```python
from build123d import *

# Parameters (mm, degrees)
F1_DEPTH = 70
F2_DEPTH = 2
F4_DEPTH = 25
F5_W     = 61
F5_H     = 2
F5_W_2   = 2
F6_DEPTH = 25


with BuildPart() as f1:
    # F0 (on Front) → F1 (new body)
    with BuildSketch(Plane.XZ):
        with BuildLine():
            Line((56, 11), (0, 11))
            ThreePointArc((0, 11), (-11, 0), (0, -11))
            Line((0, -11), (56, -11))
            ThreePointArc((56, -11), (67, 0), (56, 11))
        make_face()
        with BuildLine():
            ThreePointArc((0, -9.5), (-9.5, 0), (0, 9.5))
            Line((0, 9.5), (56, 9.5))
            ThreePointArc((56, 9.5), (65.5, 0), (56, -9.5))
            Line((56, -9.5), (0, -9.5))
        make_face(mode=Mode.SUBTRACT)
    extrude(amount=F1_DEPTH)

    # F0 (on Front) → F2 (join)
    with BuildSketch(Plane.XZ):
        with BuildLine():
            Line((56, 9.5), (0, 9.5))
            ThreePointArc((0, 9.5), (-9.5, 0), (0, -9.5))
            Line((0, -9.5), (56, -9.5))
            ThreePointArc((56, -9.5), (65.5, 0), (56, 9.5))
        make_face()
    extrude(amount=F2_DEPTH)

    # F3 (on face) → F4 (cut)
    with BuildSketch(Plane(origin=(0, 0, -11), x_dir=(1, 0, 0), z_dir=(0, 0, -1))):
        with BuildLine():
            Line((67, 70), (56, 70))
            Line((56, 70), (56, 68))
            ThreePointArc((56, 68), (59.221825, 60.221825), (67, 57))
            Line((67, 57), (67, 70))
        make_face()
    extrude(amount=-F4_DEPTH, mode=Mode.SUBTRACT)

    # F5 (on face) → F6 (cut)
    with BuildSketch(Plane(origin=(0, 0, -11), x_dir=(1, 0, 0), z_dir=(0, 0, -1))):
        with Locations((17.5, 36)):
            Rectangle(F5_W, F5_H)
        with Locations((67, 36)):
            Rectangle(F5_W_2, F5_H)
    extrude(amount=-F6_DEPTH, mode=Mode.SUBTRACT)


solid = f1.part
```
CAD build for the part. Positions are in the model's coordinates, mm. A direction names the side the tool comes from. Round coordinates to 2 decimals unless told otherwise and drop trailing zeros. Write each loop counter-clockwise with the first axis right and the second up, starting at its lowest first coordinate (ties: lowest second). Pieces come first, ordered by that corner, then holes. Notation, with made-up numbers: (11.25, 53) - (43.25, 53) arc R14 cw to (43.25, 78) - close; hole circle Ø8 at (76.5, 52.25). An arc over 180 degrees is marked (long way). Return JSON: item names as keys, results as strings. Group by question number.
Item 1: Probe probe 1 along Z at (x, y) = (40.5, -57); probe 2 along Y at (x, z) = (4, -9.75); probe 3 along Y at (x, z) = (36, -6.25). List the from-to ranges inside material, lowest first.
Item 2: Band-saw the part on C-C on y = -20. List the corners of the cut face in (x, z), plus the area to 3 significant figures.
Item 3: 3-axis set-ups, long thin cutter, end or side, ignore diameter. For faces 1 (the face through (66, -36, 0)), 2 (the face through (16, -35, -10)), 3 (the face through (-9.498, -18.269, -0.209)): which of +Z, -Z, +X, -X, +Y, -Y reach the whole face in a straight line?
Item 4: Band-saw the part on B-B on z = -7.25. List the corners of the cut face in (x, y).
Item 5: Band-saw the part on D-D on x = 51. List the corners of the cut face in (y, z), plus the area to 3 significant figures.
Item 6: Band-saw the part on A-A on x = 19. List the corners of the cut face in (y, z), plus the area to 3 significant figures.
Item 7: Mould opens along Z. For faces 4 (the face through (20, -70, 10)), 5 (the face through (-11, -53, 0)), 6 (the face through (28.4, -34.5, 11)), 7 (the face through (-9.498, -53.269, -0.209)) say: +Z half, -Z half, draft (parallel to the pull), parting line (faces both ways), or undercut.
Item 8: Flat gauge pins, fed straight in: pin 1 Ø0.8 at (y, z) = (-35.5, -10) entering from -X; pin 2 Ø5 at (y, z) = (-62.5, 8) entering from +X; pin 3 Ø5 at (y, z) = (-28.5, 8) entering from -X. Where does each tip first touch, or does it go through?
Resolved:
{
 "1": {"probe 1": "z = -11 to -9.5, 9.5 to 11", "probe 2": "y = -70 to -37, -35 to 0", "probe 3": "y = -2 to 0"},
 "2": {"outline": "(0, -11) - (56, -11) arc R11 ccw to (56, 11) - (0, 11) arc R11 ccw to start; hole (0, -9.5) - (56, -9.5) arc R9.5 ccw to (56, 9.5) - (0, 9.5) arc R9.5 ccw to start", "area": "265 mm²"},
 "3": {"face 1": "+Z, -Z, +X", "face 2": "+Z, -Z, -X", "face 3": "-Y"},
 "4": {"outline": "(-8.27, -70) - (-6.14, -70) - (-6.14, -37) - (-8.27, -37) - close; (-8.27, -35) - (-6.14, -35) - (-6.14, -2) - (62.14, -2) - (62.14, -58.13) arc R11 cw to (64.27, -57.34) - (64.27, 0) - (-8.27, 0) - close"},
 "5": {"outline": "(-70, -11) - (0, -11) - (0, 11) - (-70, 11) - (-70, 9.5) - (-2, 9.5) - (-2, -9.5) - (-70, -9.5) - close", "area": "248 mm²"},
 "6": {"outline": "(-70, -11) - (-37, -11) - (-37, -9.5) - (-70, -9.5) - close; (-70, 9.5) - (-37, 9.5) - (-37, 11) - (-70, 11) - close; (-35, -11) - (0, -11) - (0, 11) - (-35, 11) - (-35, 9.5) - (-2, 9.5) - (-2, -9.5) - (-35, -9.5) - close", "area": "242 mm²"},
 "7": {"face 4": "draft", "face 5": "parting line", "face 6": "+Z half", "face 7": "undercut"},
 "8": {"pin 1": "stops at x = 48", "pin 2": "stops at x = 59.27", "pin 3": "stops at x = -9.53"}
}
